Part model, mm, in its own coordinate system. A direction names the side the tool comes from. Round coordinates to 2 decimals unless told otherwise and drop trailing zeros. Write each loop counter-clockwise with the first axis right and the second up, starting at its lowest first coordinate (ties: lowest second). Pieces come first, ordered by that corner, then holes. Notation, with made-up numbers: M 25,73 L 33,73 A23 cw 33,88 Z; hole C 5.5,-11.5 d11. An arc over 180 degrees is marked long. Use a Markdown table: item, result. Add a question column.
1) Slice it at C-C on z = 62. Write the cut outline in (x, y), plus the area to 3 significant figures.
2) Slice it at A-A on z = 35.5. Write the cut outline in (x, y), plus the area to 3 significant figures.
3) Wall check: probe 1 along X at (y, z) = (33.3, 22.5); probe 2 along X at (y, z) = (30, 12); probe 3 along Y at (x, z) = (33, 10). Give the ranges that are in metal, low to high.
4) Drop flat-ended pins along their axis: P1, Ø5, axis at y = 26, z = 54.5, coming from the +X side; P2, Ø3.5, axis at x = 44, y = 34, coming from the -Z side; P3, Ø2.5, axis at y = 34.5, z = 38.5, coming from the +X side; P4, Ø3, axis at x = 26.5, y = 21.5, coming from the -Z side. Give the stop position or say it passes through.
5) Two-plate mould, pull along Z, no slides. Class faces 1 (the face through (44, 34, 20)), 2 (the face through (18.165, 6.069, 35.49)), 3 (the face through (24.53, 17.74, 56.45)): released by +Z, released by -Z, zero draft, split by the parting line, or undercut.
6) Which spindle directions (+Z, -Z, +X, -X, +Y, -Y) get a long thin tool onto all of the face, cutting with end or side? Do faces 4 (the face through (41.37, 34.02, 25.57)), 5 (the face through (43, 32.498, 22)), 6 (the face through (28, 21, 15.5)). Say none if no direction does.
7) Slice it at B-B on x = 42. Write the cut outline in (y, z), plus the area to 3 significant figures.
```python
from build123d import *

# Parameters (mm, degrees)
SKETCH_1_W          = 7
SKETCH_1_H          = 3
EXTRUDE_1_DEPTH     = 70
SKETCH_2_R          = 1.75
CUT_EXTRUDE_1_DEPTH = 70
SKETCH_3_W          = 7
SKETCH_3_H          = 20
CUT_EXTRUDE_2_DEPTH = 70
FILLET_1_R          = 2
FILLET_3_R          = 2
FILLET_4_R          = 2
FILLET_5_R          = 2
SKETCH_4_W          = 20
SKETCH_4_H          = 3
CUT_EXTRUDE_3_DEPTH = 7
FILLET_6_R          = 2
FILLET_7_R          = 0.5
SKETCH_5_W          = 53
SKETCH_5_H          = 18.5
CUT_EXTRUDE_4_DEPTH = 8
SKETCH_7_R          = 1.75
EXTRUDE_3_DEPTH     = 2.121320344
FILLET_9_R          = 1


with BuildPart() as part:
    # 草图1 → 凸台-拉伸1 (new body)
    with BuildSketch(Plane.XY):
        with Locations((44.266038526, 33.998202963)):
            Rectangle(SKETCH_1_W, SKETCH_1_H)
        Polygon((40.766038526, 32.498202963), (40.766038526, 35.498202963), (10.766038526, 5.498202963), (13.766038526, 5.498202963), (18.766038526, 10.498202963), align=None)
        Polygon((18.766038526, 5.498202963), (18.766038526, 10.498202963), (13.766038526, 5.498202963), align=None)
    extrude(amount=EXTRUDE_1_DEPTH)

    # 草图2 → 切除-拉伸1 (cut)
    with BuildSketch(Plane(origin=(0, 35.498202963, 0), x_dir=(1, 0, 0), z_dir=(0, 1, 0))):
        with Locations(Location((45.266038526, -22.5, 0), (0, 0, 270))):
            Circle(SKETCH_2_R)
        with Locations(Location((45.266038526, -47.5, 0), (0, 0, 270))):
            Circle(SKETCH_2_R)
    extrude(amount=-CUT_EXTRUDE_1_DEPTH, mode=Mode.SUBTRACT)

    # 草图3 → 切除-拉伸2 (cut)
    with BuildSketch(Plane(origin=(0, 35.498202963, 0), x_dir=(1, 0, 0), z_dir=(0, 1, 0))):
        with Locations((44.266038526, -10)):
            Rectangle(SKETCH_3_W, SKETCH_3_H)
        with Locations((44.266038526, -60)):
            Rectangle(SKETCH_3_W, SKETCH_3_H)
    extrude(amount=-CUT_EXTRUDE_2_DEPTH, mode=Mode.SUBTRACT)

    # 圆角1
    fillet_1_edges = [part.edges().sort_by_distance(p)[0] for p in [
        (40.766038526, 33.998202963, 20),
        (40.766038526, 33.998202963, 50),
    ]]
    fillet(fillet_1_edges, radius=FILLET_1_R)

    # 圆角3
    fillet_3_edges = [part.edges().sort_by_distance(p)[0] for p in [
        (40.766038526, 33.998202963, 0),
        (40.766038526, 33.998202963, 70),
    ]]
    fillet(fillet_3_edges, radius=FILLET_3_R)

    # 圆角4
    fillet_4_edges = [part.edges().sort_by_distance(p)[0] for p in [
        (18.766038526, 10.498202963, 35),
        (18.766038526, 5.498202963, 35),
    ]]
    fillet(fillet_4_edges, radius=FILLET_4_R)

    # 圆角5
    fillet_5_edges = [part.edges().sort_by_distance(p)[0] for p in [
        (47.766038526, 33.998202963, 20),
        (47.766038526, 33.998202963, 50),
    ]]
    fillet(fillet_5_edges, radius=FILLET_5_R)

    # 草图4 → 切除-拉伸3 (cut)
    with BuildSketch(Plane(origin=(47.766038526, 0, 0), x_dir=(0, 0, -1), z_dir=(1, 0, 0))):
        with Locations((-35, 33.998202963)):
            Rectangle(SKETCH_4_W, SKETCH_4_H)
    extrude(amount=-CUT_EXTRUDE_3_DEPTH, mode=Mode.SUBTRACT)

    # 圆角6
    fillet_6_edges = [part.edges().sort_by_distance(p)[0] for p in [
        (40.766038526, 33.998202963, 45),
        (40.766038526, 33.998202963, 25),
        (47.766038526, 33.998202963, 45),
        (47.766038526, 33.998202963, 25),
    ]]
    fillet(fillet_6_edges, radius=FILLET_6_R)

    # 圆角7
    fillet_7_edges = [part.edges().sort_by_distance(p)[0] for p in [
        (10.766038526, 5.498202963, 35),
    ]]
    fillet(fillet_7_edges, radius=FILLET_7_R)

    # 草图5 → 切除-拉伸4 (cut)
    with BuildSketch(Plane(origin=(2.633917782, -2.633917782, 0), x_dir=(0, 0, 1), z_dir=(-0.7071067811865477, 0.7071067811865475, 0))):
        with Locations((35, 34.676962319)):
            Rectangle(SKETCH_5_W, SKETCH_5_H)
    extrude(amount=-CUT_EXTRUDE_4_DEPTH, mode=Mode.SUBTRACT)

    # 草图7 → 凸台-拉伸3 (add)
    # profile 1 of 2: a face of its own
    with BuildSketch(Plane(origin=(2.633917782, -2.633917782, 0), x_dir=(0, 0, 1), z_dir=(-0.7071067811865477, 0.7071067811865475, 0))):
        Polygon((13.25, 39.176962319), (15.5, 39.176962319), (15.5, 30.176962319), (13.25, 30.176962319), (13.25, 25.426962319), (8.5, 25.426962319), (8.5, 43.926962319), (13.25, 43.926962319), align=None)
        with Locations(Location((12.5, 34.676962319, 0), (0, 0, 270))):
            Circle(SKETCH_7_R, mode=Mode.SUBTRACT)
    # profile 2 of 2: a face of its own
    with BuildSketch(Plane(origin=(2.633917782, -2.633917782, 0), x_dir=(0, 0, 1), z_dir=(-0.7071067811865477, 0.7071067811865475, 0))):
        Polygon((56.75, 30.176962319), (54.5, 30.176962319), (54.5, 39.176962319), (56.75, 39.176962319), (56.75, 43.926962319), (61.5, 43.926962319), (61.5, 35.176962319), (61.5, 25.426962319), (56.75, 25.426962319), align=None)
        with Locations(Location((57.5, 34.676962319, 0), (0, 0, 270))):
            Circle(SKETCH_7_R, mode=Mode.SUBTRACT)
    extrude(amount=-EXTRUDE_3_DEPTH)

    # 圆角9
    fillet_9_edges = [part.edges().sort_by_distance(p)[0] for p in [
        (34.444970714, 27.677135151, 13.25),
        (31.086213504, 24.31837794, 13.25),
        (31.086213504, 24.31837794, 15.5),
        (24.722252473, 17.954416909, 15.5),
        (24.722252473, 17.954416909, 13.25),
        (21.363495262, 14.595659699, 13.25),
        (21.363495262, 14.595659699, 56.75),
        (24.722252473, 17.954416909, 56.75),
        (24.722252473, 17.954416909, 54.5),
        (31.086213504, 24.31837794, 54.5),
        (31.086213504, 24.31837794, 56.75),
        (34.444970714, 27.677135151, 56.75),
    ]]
    fillet(fillet_9_edges, radius=FILLET_9_R)


solid = part.part
```
Entries:
| question | item | result |
|---|---|---|
| 1 | outline | M 11.62,6.35 A0.5 ccw 11.97,5.5 L 16.77,5.5 A2 ccw 18.77,7.5 L 18.77,9.67 A2 cw 19.35,11.08 L 40.77,32.5 L 40.77,35.5 Z |
| 1 | area | 96.9 mm^2 |
| 2 | outline | M 11.62,6.35 A0.5 ccw 11.97,5.5 L 16.77,5.5 A2 ccw 18.77,7.5 L 18.77,9.67 A2 cw 19.35,11.08 L 22.11,13.85 L 20.61,15.35 Z; M 33.69,28.43 L 35.19,26.93 L 40.77,32.5 L 40.77,35.5 Z |
| 2 | area | 57.7 mm^2 |
| 3 | probe 1 | x = 38.57 to 43.52, 47.02 to 47.77 |
| 3 | probe 2 | x = 35.27 to 38.27 |
| 3 | probe 3 | y = 24.73 to 27.73 |
| 4 | P1 | stops at x = 36.77 |
| 4 | P2 | stops at z = 19.93 |
| 4 | P3 | stops at x = 40.77 |
| 4 | P4 | stops at z = 0 |
| 5 | face 1 | released by -Z |
| 5 | face 2 | zero draft |
| 5 | face 3 | undercut |
| 6 | face 4 | +X, +Y, -Y |
| 6 | face 5 | +Z, -Z, +X, -Y |
| 6 | face 6 | +X, -X, +Y, -Y |
| 7 | outline | M 32.5,19.85 L 35.5,19.85 L 35.5,25.15 L 32.5,25.15 Z; M 32.5,44.85 L 35.5,44.85 L 35.5,50.15 L 32.5,50.15 Z |
| 7 | area | 31.8 mm^2 |
